from build123d import *
from build123d.topology import SkipClean

# Parameters (mm, degrees)
BASPROSKE_W      = 8
BASPROSKE_H      = 8.5
TOOTHCUT_DEPTH   = 15.439529078
TEETHCUTS_COUNT  = 15
TEETHCUTS_ANGLE  = 336
HUBNEAONESKE_R   = 6.249
HUBNEARONE_DEPTH = 3.0001524
BORSKE_R         = 3
BORE_DEPTH       = 11.0001524
MOVE_FACE1_BY    = 3


with BuildPart() as part:
    # BasProSke → Base-Revolve (revolve)
    with BuildSketch(Plane(origin=(0, 0, 0), x_dir=(1, 0, 0), z_dir=(0, 1, 0)), mode=Mode.PRIVATE) as base_revolve_sk:
        with Locations((4, 4.25)):
            Rectangle(BASPROSKE_W, BASPROSKE_H)
    revolve(base_revolve_sk.sketch.rotate(Axis((-10, 0, 0), (1, 0, 0)), 180), axis=Axis((-10, 0, 0), (1, 0, 0)))

    # TooCutSke → ToothCut (cut, through all)
    with BuildSketch(Plane(origin=(0, 0, 0), x_dir=(0, 0, -1), z_dir=(1, 0, 0))):
        with BuildLine():
            ThreePointArc((0.531576138, 6.226349477), (0, 6.249), (-0.531576138, 6.226349477))
            ThreePointArc((-0.531576138, 6.226349477), (-0.830301624, 7.411024729), (-1.576608494, 8.378350125))
            ThreePointArc((-1.576608494, 8.378350125), (0, 8.5254), (1.576608494, 8.378350125))
            ThreePointArc((1.576608494, 8.378350125), (0.830301624, 7.411024729), (0.531576138, 6.226349477))
        make_face()
    toothcut = extrude(amount=TOOTHCUT_DEPTH, mode=Mode.SUBTRACT)

    # TeethCuts: ToothCut ×15 about axis
    teethcuts_axis = Axis((-10, 0, 0), (1, 0, 0))
    for i in range(1, TEETHCUTS_COUNT):
        add(toothcut.rotate(teethcuts_axis, i * TEETHCUTS_ANGLE / (TEETHCUTS_COUNT - 1)), mode=Mode.SUBTRACT)

    # HubNeaOneSke → HubNearOne (add)
    with SkipClean():  # the faces are left unmerged after this step: merging them gives an invalid solid
        with BuildSketch(Plane.ZY):
            Circle(HUBNEAONESKE_R)
        extrude(amount=HUBNEARONE_DEPTH)

    # BorSke → Bore (cut, symmetric)
    with SkipClean():  # the faces are left unmerged after this step: merging them gives an invalid solid
        with BuildSketch(Plane(origin=(0, 0, 0), x_dir=(0, 0, -1), z_dir=(1, 0, 0))):
            with Locations(Location((0, 0, 0), (0, 0, 180))):
                Circle(BORSKE_R)
        extrude(amount=BORE_DEPTH, both=True, mode=Mode.SUBTRACT)

    # Move Face1: a face moved outward by 3.0
    extrude(part.faces().sort_by_distance((-3.0001524, -3.1245, 0))[0], amount=MOVE_FACE1_BY, dir=(-1, 0, 0))


solid = part.part
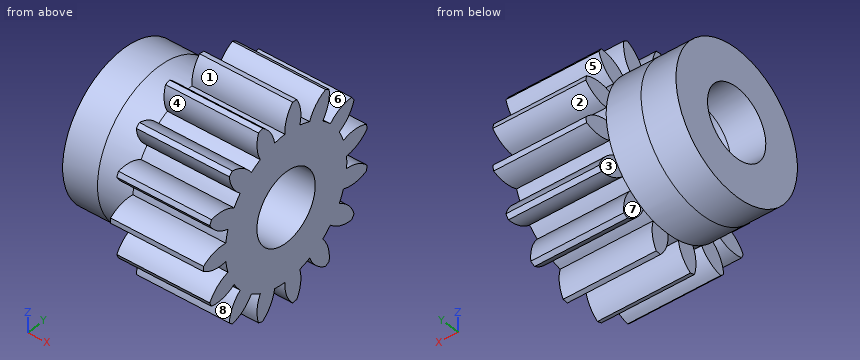
For this review, take the finished solid that the model builds, in its own axes (mm). Face numbers are marked on the shaded views. A direction names the side the tool comes from. Give positions to 0.01 mm unless a question says otherwise; leave off trailing zeros. One line per question, with ' | ' between items.
1) The part is to be moulded in two halves that separate along Y. For the marked faces 1, 2 and 3, say which applies: +Y half, -Y half, draft (parallel to the pull), parting line (faces both ways), or undercut.
Resolved:
face 1: undercut | face 2: +Y half | face 3: draft
2) Insertion check: pin 1 Ø3.5 at (y, z) = (0, 0) entering from -X. The pin has a flat end and moves straight along its axis. Give the tip position at first contact, or say it passes through.
Resolved:
pin 1: passes through
3) For the marked faces 4, 5, 6, 7 and 8, list the 3-axis set-ups (+Z, -Z, +X, -X, +Y, -Y) from which the entire face can be reached by the end or side of a thin tool; tool diameter is ignored.
Resolved:
face 4: +X, -X | face 5: +X, -X, +Y | face 6: +Z, +X, -X | face 7: -Z, -X, +Y | face 8: +X, -X, -Y
